Autodesk Inventor part; units mm, degrees
ref_plane "YZ Plane" through (0, 0, 0) normal (1, 0, 0) x (0, 1, 0)
ref_plane "XZ Plane" through (0, 0, 0) normal (0, 1, 0) x (-1, 0, 0)
ref_plane "XY Plane" through (0, 0, 0) normal (0, 0, 1) x (1, 0, 0)
sketch "Sketch1" plane through (0, 0, 0) normal (0, 0, 1) x (1, 0, 0)
  line L0 (0, 0) -> (0, 7.5)
  line L1 (0, 7.5) -> (24, 7.5)
  line L2 (24, 7.5) -> (24, 5)
  line L3 (24, 5) -> (29, 5)
  line L4 (29, 5) -> (29, 0)
  line L5 (29, 0) -> (0, 0)
  dimension "d0" = 24
  dimension "d1" = 5
  dimension "d2" = 15
  dimension "d3" = 10
revolve "Revolution1" add sketch "Sketch1" angle 360 about axis through (29, 0, 0) along (-1, 0, 0)
sketch "Sketch2" plane through (0, 0, 0) normal (-1, 0, 0) x (0, 0, 1)
  circle A0 centre (0, 0) radius 7.5
  point P0 (0, 0)
hole "Hole1" at (0, 0, 0) direction (1, 0, 0) diameter 3 depth 29 counterbore diameter 8 counterbore depth 18
thread "Thread1"
properties part number "1 part 18"
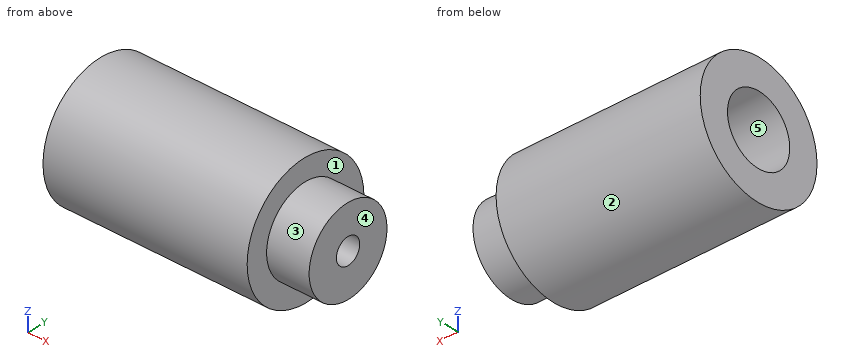
Input: part model. Units: mm. Frame: model coordinates. Face numbers are marked on the shaded views. A direction names the side the tool comes from. Coordinates: 2 decimals unless noted, no trailing zeros. Order: outer loops, then holes, each group sorted by start corner. A loop starts at its lowest first (then second) coordinate and runs counter-clockwise, first axis right, second up. Notation, with made-up numbers: (-9.5, 19) - (46.5, 19) arc R21 cw to (46.5, 39) - close; hole circle Ø11 at (85.25, -28). An arc over 180 degrees is marked (long way). Return JSON: item names as keys, results as strings.
Q1. Draft query along Z for the marked faces 3, 4 and 5. Return one class per face: +Z half, -Z half, draft (parallel to the pull), parting line (faces both ways), or undercut.
The answers:
{"face 3": "parting line", "face 4": "draft", "face 5": "undercut"}
Q2. Cut plane D-D (x = 19). Return loops of the section in (y, z), then the cut area to 3 significant figures.
The answers:
{"outline": "circle Ø15 at (0, 0); hole circle Ø3 at (0, 0)", "area": "170 mm2"}
Q3. First-contact query: pin 1 (2 mm diameter, centred on x = 12.5, z = -0.5, fed in from +Y); pin 2 (5 mm diameter, centred on y = 0, z = 0, fed in from -X); pin 3 (3 mm diameter, centred on x = 13.5, z = 2.5, fed in from +Y); pin 4 (5 mm diameter, centred on x = 10, z = 5.5, fed in from -Y). Flat tips, straight axial feed; report the tip coordinate or a pass-through.
The answers:
{"pin 1": "stops at y = 7.5", "pin 2": "stops at x = 18", "pin 3": "stops at y = 7.43", "pin 4": "stops at y = -6.87"}
Q4. Access query for the marked faces 1 and 2. Directions: +Z, -Z, +X, -X, +Y, -Y. A direction counts if a zero-diameter tool reaches every point of the face in a straight line with its end or side. Return the directions, or none.
The answers:
{"face 1": "+X", "face 2": "+X, -X"}
Q5. Cut plane C-C (y = -4.5). Return loops of the section in (x, z).
The answers:
{"outline": "(0, -6) - (24, -6) - (24, -2.18) - (29, -2.18) - (29, 2.18) - (24, 2.18) - (24, 6) - (0, 6) - close"}
Q6. Ray query, probe 1 along Z at (x, y) = (5, 0); probe 2 along Z at (x, y) = (21.75, 0). Return the intervals inside material, ascending.
The answers:
{"probe 1": "z = -7.5 to -4, 4 to 7.5", "probe 2": "z = -7.5 to -1.5, 1.5 to 7.5"}
Q7. Cut plane A-A (z = 0). Return loops of the section in (x, y).
The answers:
{"outline": "(0, -7.5) - (24, -7.5) - (24, -5) - (29, -5) - (29, -1.5) - (18, -1.5) - (18, -4) - (0, -4) - close; (0, 4) - (18, 4) - (18, 1.5) - (29, 1.5) - (29, 5) - (24, 5) - (24, 7.5) - (0, 7.5) - close"}
